Autodesk Inventor part; units mm, degrees
ref_plane "YZ Plane" through (0, 0, 0) normal (1, 0, 0) x (0, 1, 0)
ref_plane "XZ Plane" through (0, 0, 0) normal (0, 1, 0) x (-1, 0, 0)
ref_plane "XY Plane" through (0, 0, 0) normal (0, 0, 1) x (1, 0, 0)
sketch "Block1" plane through (0, 0, 0) normal (0, 0, 1) x (1, 0, 0)
  circle A0 centre (74.029, 24.2723) radius 1
  line L0 (49.279, 30.4723) -> (71.779, 30.4723)
  line L1 (71.779, 30.4723) -> (71.779, 18.0723)
  line L2 (71.779, 18.0723) -> (49.279, 18.0723)
  line L3 (49.279, 18.0723) -> (49.279, 30.4723)
  line L4 (49.279, 30.4723) -> (44.779, 30.4723)
  line L5 (44.779, 30.4723) -> (44.779, 18.0723)
  line L6 (44.779, 18.0723) -> (49.279, 18.0723)
  line L7 (49.279, 18.0723) -> (49.279, 30.4723)
  line L8 (71.779, 30.4723) -> (76.279, 30.4723)
  line L9 (76.279, 30.4723) -> (76.279, 18.0723)
  line L10 (76.279, 18.0723) -> (71.779, 18.0723)
  line L11 (71.779, 18.0723) -> (71.779, 30.4723)
  line L12 (44.779, 24.2723) -> (76.279, 24.2723) construction
  line L13 (47.029, 30.4723) -> (47.029, 18.0723) construction
  circle A1 centre (47.029, 24.2723) radius 1
  line L14 (74.029, 30.4723) -> (74.029, 18.0723) construction
  point P0 (60.979, 24.0984)
  dimension "d7" = 22.5
  dimension "d8" = 12.4
  dimension "d9" = 4.5
  dimension "d10" = 4.5
  dimension "d11" = 2
  dimension "d12" = 2
sketch "Sketch1" plane through (0, 0, 0) normal (0, 0, 1) x (1, 0, 0)
  line L0 (-92.7646, -8.503) -> (-89.7646, -8.503)
  line L1 (-89.7646, -8.503) -> (-89.7646, -11.753)
  line L2 (-89.7646, -11.753) -> (-92.7646, -11.753)
  line L3 (-92.7646, -11.753) -> (-92.7646, -8.503)
  line L4 (-92.7646, -21.6527) -> (-89.7646, -21.6527)
  line L5 (-89.7646, -21.6527) -> (-89.7646, -21.7527)
  line L6 (-89.7646, -21.7527) -> (-92.7646, -21.7527)
  line L7 (-92.7646, -21.7527) -> (-92.7646, -21.6527)
  line L8 (8.2668, 7.2563) -> (35.2668, 7.2563)
  line L9 (35.2668, 7.2563) -> (35.2668, 15.7563)
  line L10 (35.2668, 15.7563) -> (8.2668, 15.7563)
  line L11 (8.2668, 15.7563) -> (8.2668, 7.2563)
  line L12 (8.2668, 11.5063) -> (35.2668, 11.5063) construction
  line L13 (21.7668, 15.7563) -> (21.7668, 7.2563) construction
  line L14 (19.2668, 19.0063) -> (24.2668, 19.0063)
  line L15 (24.2668, 19.0063) -> (24.2668, 15.7563)
  line L16 (24.2668, 15.7563) -> (19.2668, 15.7563)
  line L17 (19.2668, 15.7563) -> (19.2668, 19.0063)
  line L18 (21.7668, 19.0063) -> (21.7668, 15.7563) construction
  line L19 (19.2668, 4.0063) -> (24.2668, 4.0063)
  line L20 (24.2668, 4.0063) -> (24.2668, 7.2563)
  line L21 (24.2668, 7.2563) -> (19.2668, 7.2563)
  line L22 (19.2668, 7.2563) -> (19.2668, 4.0063)
  line L23 (21.7668, 4.0063) -> (21.7668, 7.2563) construction
  line L24 (5.0168, 14.0063) -> (8.2668, 14.0063)
  line L25 (8.2668, 14.0063) -> (8.2668, 9.0063)
  line L26 (8.2668, 9.0063) -> (5.0168, 9.0063)
  line L27 (5.0168, 9.0063) -> (5.0168, 14.0063)
  line L28 (5.0168, 11.5063) -> (8.2668, 11.5063) construction
  line L29 (38.5168, 14.0063) -> (35.2668, 14.0063)
  line L30 (35.2668, 14.0063) -> (35.2668, 9.0063)
  line L31 (35.2668, 9.0063) -> (38.5168, 9.0063)
  line L32 (38.5168, 9.0063) -> (38.5168, 14.0063)
  line L33 (38.5168, 11.5063) -> (35.2668, 11.5063) construction
  point P0 (0, 0)
  point P1 (21.7668, 4.0063)
  dimension "d0" = 3
  dimension "mat" = 3.25
  dimension "d2" = 3
  dimension "d3" = 0.1
  dimension "d58" = 27
  dimension "d59" = 8.5
  dimension "d62" = 5
  dimension "d63" = 3.25
  dimension "d64" = 3.25
  dimension "d65" = 5
extrude "Extrusion5" add sketch "Sketch1" along normal blind 3.25 contours L11 L10 L9 L8
extrude "Extrusion6" cut sketch "Sketch1" along normal blind 3.25 contours L8 L20 L19 L22 | L26 L27 L24 L11 | L9 L29 L32 L31 | L17 L14 L15 L10
extrude "Extrusion7" add sketch "Sketch1" along normal blind 3.25 contours L26 L27 L24 L11 | L9 L29 L32 L31
extrude "Extrusion8" add sketch "Sketch1" along normal blind 3.25 contours L8 L20 L19 L22 | L17 L14 L15 L10
equation "\"d63\" = mat"
equation "\"d64\" = mat"
equation "\"d60\" = mat"
equation "\"d66\" = mat"
equation "\"d68\" = mat"
equation "\"d70\" = mat"
properties part number "arm-servo"
For this review, take the finished solid that the model builds, in its own axes (mm). A direction names the side the tool comes from. Coordinates: 2 decimals unless noted, no trailing zeros. Write each loop counter-clockwise with the first axis right and the second up, starting at its lowest first coordinate (ties: lowest second). Pieces come first, ordered by that corner, then holes. Notation, with made-up numbers: (68, 87.25) - (79, 87.25) arc R15 ccw to (79, 106.25) - close; hole circle Ø1 at (35, 54.25). An arc over 180 degrees is marked (long way). Answer in a Markdown table with one row per item. Add a question column.
Q1. We need section B-B, the plane x = 32. State the section outline as (y, z) points.
Q2. We need section C-C, the plane y = 6.25. State the section outline as (x, z) points, and give its area (4 significant figures).
Q3. For P1, Ø1.6, axis at x = 37, z = 1, coming from the +Y side; P2, Ø0.5, axis at y = 8, z = 1.5, coming from the +X side; P3, Ø1.6, axis at x = 37, z = 1.5, coming from the -Y side, all flat-tipped, find the tip position at first contact; note any pin that passes through.
Q4. Tool access review of faces 1 (the flat face through (30, 7.256, 2)), 2 (the flat face through (22, 19.006, 2)), 3 (the flat face through (7, 14.006, 2)), 4 (the flat face through (19.267, 6, 2)), 5 (the flat face through (37, 14.006, 2)): name each direction out of +Z, -Z, +X, -X, +Y, -Y from which nothing blocks a thin tool from reaching the whole face with its end or side.
Q5. For probe 1 along Y at (x, z) = (27, 0.4); probe 2 along X at (y, z) = (18.25, 3); probe 3 along X at (y, z) = (8, 2.05), list the stretches that pass through material, from the lowest coordinate up.
Q6. We need section A-A, the plane z = 1.65. State the section outline as (x, y) points.
Answer list:
| question | item | result |
|---|---|---|
| 1 | outline | (7.26, 0) - (15.76, 0) - (15.76, 3.25) - (7.26, 3.25) - close |
| 2 | outline | (19.27, 0) - (24.27, 0) - (24.27, 3.25) - (19.27, 3.25) - close |
| 2 | area | 16.25 mm2 |
| 3 | P1 | stops at y = 14.01 |
| 3 | P2 | stops at x = 35.27 |
| 3 | P3 | stops at y = 9.01 |
| 4 | face 1 | +Z, -Z, +X, -Y |
| 4 | face 2 | +Z, -Z, +X, -X, +Y |
| 4 | face 3 | +Z, -Z, -X, +Y |
| 4 | face 4 | +Z, -Z, -X, -Y |
| 4 | face 5 | +Z, -Z, +X, +Y |
| 5 | probe 1 | y = 7.26 to 15.76 |
| 5 | probe 2 | x = 19.27 to 24.27 |
| 5 | probe 3 | x = 8.27 to 35.27 |
| 6 | outline | (5.02, 9.01) - (8.27, 9.01) - (8.27, 7.26) - (19.27, 7.26) - (19.27, 4.01) - (24.27, 4.01) - (24.27, 7.26) - (35.27, 7.26) - (35.27, 9.01) - (38.52, 9.01) - (38.52, 14.01) - (35.27, 14.01) - (35.27, 15.76) - (24.27, 15.76) - (24.27, 19.01) - (19.27, 19.01) - (19.27, 15.76) - (8.27, 15.76) - (8.27, 14.01) - (5.02, 14.01) - close |
